Part model, mm, in its own coordinate system. Face numbers are marked on the shaded views. Give positions to 0.01 mm unless a question says otherwise; leave off trailing zeros. Write each loop counter-clockwise with the first axis right and the second up, starting at its lowest first coordinate (ties: lowest second). Pieces come first, ordered by that corner, then holes. Notation, with made-up numbers: (-4, -23) - (33, -23) arc R34 ccw to (33, 7) - close; hole circle Ø3 at (61.25, 32.25). An arc over 180 degrees is marked (long way). Answer in a Markdown table with one row per item. Add a question column.
1. Pull direction X, two halves, no side cores. Call the marked faces 1, 2 and 3: released by +X, released by -X, zero draft, split by the parting line, or undercut.
2. Band-saw the part on B-B on z = -1. Write the cut outline in (x, y).
3. Band-saw the part on D-D on z = -13. Write the cut outline in (x, y).
4. Drop flat-ended pins along their axis: pin 1 Ø3 at (y, z) = (-6.5, -1.5) entering from -X; pin 2 Ø6 at (x, y) = (13.5, -0.5) entering from -Z; pin 3 Ø4 at (y, z) = (-1, -13) entering from -X; pin 4 Ø3 at (x, y) = (14, 7.5) entering from +Z. Give the stop position or say it passes through.
5. Probe line 1 along X through (y, z) = (-10.5, -12.5); line 2 along X through (y, z) = (5.25, -9); line 3 along X through (y, z) = (2.25, 3). List the from-to ranges inside material, lowest first.
6. Band-saw the part on C-C on y = -2.75. State how many separate pieces and enclosed holes the cut face has, plus the area to 3 significant figures.
```python
from build123d import *

# Parameters (mm, degrees)
F0_R     = 3.175
F0_R_2   = 1.5875
F1_DEPTH = 12.7


with BuildPart() as f1:
    # F0 (on Front) → F1 (new body, symmetric)
    with BuildSketch(Plane.XZ):
        with BuildLine():
            ThreePointArc((-14.9178970331, 11.8473139618), (-8.248891971, 4.7625), (-17.7190233741, 6.9956208208))
            ThreePointArc((-17.7190233741, 6.9956208208), (-16.4977839421, -9.525), (-2.801126341, -18.8429347826))
            ThreePointArc((-2.801126341, -18.8429347826), (0, -9.525), (2.801126341, -18.8429347826))
            ThreePointArc((2.801126341, -18.8429347826), (16.4977839421, -9.525), (17.7190233741, 6.9956208208))
            ThreePointArc((17.7190233741, 6.9956208208), (8.248891971, 4.7625), (14.9178970331, 11.8473139618))
            ThreePointArc((14.9178970331, 11.8473139618), (0, 19.05), (-14.9178970331, 11.8473139618))
        make_face()
        with Locations((-9.228419212, -11.1939090512)):
            Circle(F0_R, mode=Mode.SUBTRACT)
        with Locations((-14.308419212, -2.3950909488)):
            Circle(F0_R, mode=Mode.SUBTRACT)
        with Locations((9.228419212, -11.1939090512)):
            Circle(F0_R, mode=Mode.SUBTRACT)
        Circle(F0_R_2, mode=Mode.SUBTRACT)
        with Locations((14.308419212, -2.3950909488)):
            Circle(F0_R, mode=Mode.SUBTRACT)
        with Locations((-5.08, 13.589)):
            Circle(F0_R, mode=Mode.SUBTRACT)
        with Locations((5.08, 13.589)):
            Circle(F0_R, mode=Mode.SUBTRACT)
    extrude(amount=F1_DEPTH, both=True)


solid = f1.part
```
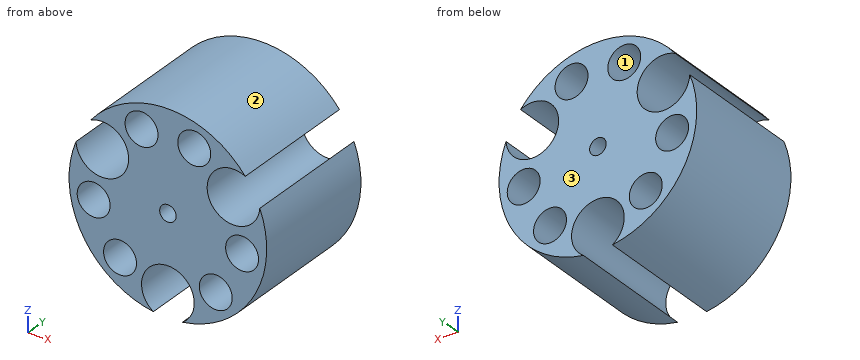
Values:
| question | item | result |
|---|---|---|
| 1 | face 1 | undercut |
| 1 | face 2 | split by the parting line |
| 1 | face 3 | zero draft |
| 2 | outline | (-19.02, -12.7) - (-17.16, -12.7) - (-17.16, 12.7) - (-19.02, 12.7) - close; (-11.46, -12.7) - (-1.23, -12.7) - (-1.23, 12.7) - (-11.46, 12.7) - close; (1.23, -12.7) - (11.46, -12.7) - (11.46, 12.7) - (1.23, 12.7) - close; (17.16, -12.7) - (19.02, -12.7) - (19.02, 12.7) - (17.16, 12.7) - close |
| 3 | outline | (-13.92, -12.7) - (-11.84, -12.7) - (-11.84, 12.7) - (-13.92, 12.7) - close; (-6.62, -12.7) - (-4.82, -12.7) - (-4.82, 12.7) - (-6.62, 12.7) - close; (4.82, -12.7) - (6.62, -12.7) - (6.62, 12.7) - (4.82, 12.7) - close; (11.84, -12.7) - (13.92, -12.7) - (13.92, 12.7) - (11.84, 12.7) - close |
| 4 | pin 1 | stops at x = -19.05 |
| 4 | pin 2 | stops at z = -15.9 |
| 4 | pin 3 | stops at x = -15.55 |
| 4 | pin 4 | stops at z = 14.38 |
| 5 | line 1 | x = -14.38 to -12.12, -6.33 to -4.62, 4.62 to 6.33, 12.12 to 14.38 |
| 5 | line 2 | x = -16.79 to -11.52, -6.93 to 6.93, 11.52 to 16.79 |
| 5 | line 3 | x = -18.81 to -15.35, -9.95 to 9.95, 15.35 to 18.81 |
| 6 | separate pieces | 1 |
| 6 | enclosed holes | 7 |
| 6 | area | 706 mm² |
